Input: part model. Units: mm. Frame: model coordinates. A direction names the side the tool comes from. Coordinates: 2 decimals unless noted, no trailing zeros. Loops run counter-clockwise (first coordinate to the right, second up) from the corner with the lowest first, then second, coordinate; pieces in that order, holes last. Notation, with made-up numbers: (75, 54) -> (123, 54) arc R18 cw to (123, 83) -> close; hole circle Ø5 at (11.5, 85). An arc over 180 degrees is marked (long way). Put each result on its own line as item: value. Start each with the question number.
1) Material intervals for L1, parallel to Y at x = 3.75, z = 0; L2, parallel to Y at x = -3, z = 0; L3, parallel to X at y = 2.5, z = -4.5, sorted ascending.
2) Set-up query: faces 1 (the flat face through (7.62, 0, -3)), 2 (the flat face through (0, -2, 5)). Return all of +Z, -Z, +X, -X, +Y, -Y with unobstructed straight access to the full face (end or side cutting, diameter ignored); none if empty.
3) Cut plane A-A (z = 0). Return the cut outline in (x, y).
4) Pull-direction query (Y, two-part tool) for faces 3 (the flat face through (-6.858, 3, 2)), 4 (the flat face through (0, 0, -2.654)), 5 (the cylindrical face through (0.28, 0.115, 3.252)), 6 (the cylindrical face through (3.757, 5.037, 0.661)); classes: pulls with the +Y half, pulls with the -Y half, needs draft (parallel to the pull), parting line crosses it, or undercut.
5) Contact query for flat-ended pins moving along their axis: P1, Ø1.5, axis at y = -3, z = -1, coming from the +X side; P2, Ø3, axis at y = -6.5, z = 6.5, coming from the +X side; P3, Ø3, axis at x = -4, z = 2.5, coming from the +Y side; P4, Ø1.1, axis at x = 1, y = 0, coming from the +Z side. Output: stop coordinate, or through.
6) Cut plane C-C (x = 5). Return the cut outline in (y, z).
7) Cut plane D-D (y = -8.25). Return the cut outline in (x, z).
8) Cut plane B-B (y = 0). Return the cut outline in (x, z).
from build123d import *

# Parameters (mm, degrees)
SKETCH1_R           = 5.08
BOSS_EXTRUDE1_DEPTH = 7.62
SKETCH2_R           = 10.9855
BOSS_EXTRUDE2_DEPTH = 6.858
CUT_EXTRUDE1_REACH  = 16.478


with BuildPart() as part:
    # Sketch1 → Boss-Extrude1 (new body)
    with BuildSketch(Plane(origin=(0, 0, 0), x_dir=(0, 0, -1), z_dir=(1, 0, 0))):
        Circle(SKETCH1_R)
    extrude(amount=BOSS_EXTRUDE1_DEPTH)

    # Sketch2 → Boss-Extrude2 (add)
    with BuildSketch(Plane.ZY):
        Circle(SKETCH2_R)
    extrude(amount=BOSS_EXTRUDE2_DEPTH)

    # Sketch3 → Cut-Extrude1 (cut, up to next)
    with BuildSketch(Plane.ZY.offset(6.858), mode=Mode.PRIVATE) as cut_extrude1_sk1:
        with BuildLine():
            Line((-2.654, -1.882763926), (-2.654, 1.882763926))
            ThreePointArc((-2.654, 1.882763926), (3.254, 0), (-2.654, -1.882763926))
        make_face()
    cut_extrude1_tool1 = extrude(cut_extrude1_sk1.sketch, amount=-CUT_EXTRUDE1_REACH, mode=Mode.PRIVATE) & part.part
    add(cut_extrude1_tool1.solids().sort_by_distance((-6.858, 0, 0.140232))[0], mode=Mode.SUBTRACT)


solid = part.part
Results found:
1. L1: y = -5.08 to -3.25, 3.25 to 5.08
1. L2: y = -10.99 to -3.25, 3.25 to 10.99
1. L3: x = -6.86 to 0
2. face 1: +Z, -Z, +X, +Y, -Y
2. face 2: +X
3. outline: (-6.86, -10.99) -> (0, -10.99) -> (0, -5.08) -> (7.62, -5.08) -> (7.62, -3.25) -> (-6.86, -3.25) -> close; (-6.86, 3.25) -> (7.62, 3.25) -> (7.62, 5.08) -> (0, 5.08) -> (0, 10.99) -> (-6.86, 10.99) -> close
4. face 3: needs draft
4. face 4: undercut
4. face 5: undercut
4. face 6: parting line crosses it
5. P1: stops at x = 7.62
5. P2: stops at x = 0
5. P3: stops at y = 10.94
5. P4: stops at z = 5.08
6. outline: circle Ø10.16 at (0, 0); hole (-1.88, -2.65) -> (1.88, -2.65) arc R3.25 ccw (long way) to start
7. outline: (-6.86, -7.25) -> (0, -7.25) -> (0, 7.25) -> (-6.86, 7.25) -> close
8. outline: (-6.86, -10.99) -> (0, -10.99) -> (0, -5.08) -> (7.62, -5.08) -> (7.62, -2.65) -> (-6.86, -2.65) -> close; (-6.86, 3.25) -> (7.62, 3.25) -> (7.62, 5.08) -> (0, 5.08) -> (0, 10.99) -> (-6.86, 10.99) -> close
